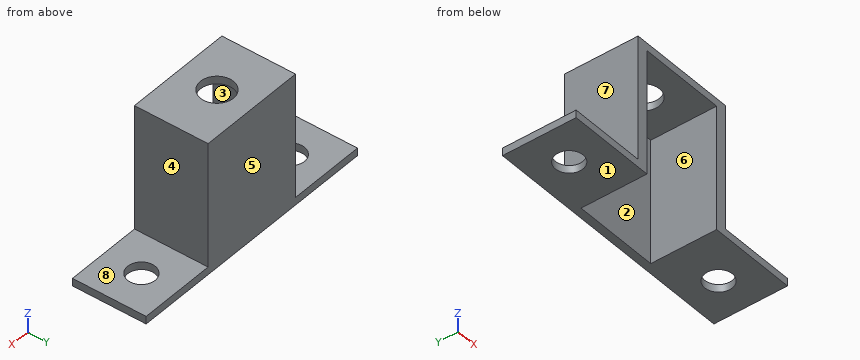
from build123d import *

# Parameters (mm, degrees)
F0_W     = 17.78
F0_H     = 1.778
F1_DEPTH = 17.018
F0_W_2   = 19.9898
F0_H_2   = 28.956
F2_DEPTH = 1.778
F5_R     = 3.175
F4_R     = 3.175
F3_R     = 3.81
F6_DEPTH = 25.4


with BuildPart() as f1:
    # F0 (on Front) → F1 (new body)
    with BuildSketch(Plane.XZ):
        Polygon((-12.296648, -10.522948), (-12.296648, -12.300948), (-9.756648, -12.300948), (-9.756648, 16.655052), (10.233152, 16.655052), (10.233152, -12.300948), (12.773152, -12.300948), (12.773152, -10.522948), (12.773152, 18.433052), (-12.296648, 18.433052), align=None)
        with Locations((-21.186648, -11.411948)):
            Rectangle(F0_W, F0_H)
        with Locations((21.663152, -11.411948)):
            Rectangle(F0_W, F0_H)
    extrude(amount=F1_DEPTH)

    # F0 (on Front) → F2 (join)
    with BuildSketch(Plane.XZ):
        with Locations((0.238252, 2.177052)):
            Rectangle(F0_W_2, F0_H_2)
    extrude(amount=F2_DEPTH)

    # F5 (on face) + F4 (on face) + F3 (on face) → F6 (cut)
    with BuildSketch(Plane.XY.offset(-10.522948)):
        with Locations((21.663152, -8.255)):
            Circle(F5_R)
    with BuildSketch(Plane.XY.offset(-10.522948)):
        with Locations((-21.186648, -8.255)):
            Circle(F4_R)
    with BuildSketch(Plane.XY.offset(18.433052)):
        with Locations((0, -8.251561)):
            Circle(F3_R)
    extrude(amount=-F6_DEPTH, mode=Mode.SUBTRACT)


solid = f1.part
Work out the finished part from the listing and answer in its coordinate system (mm). Face numbers are marked on the shaded views. A direction names the side the tool comes from. Give positions to 0.01 mm unless a question says otherwise; leave off trailing zeros. Loops run counter-clockwise (first coordinate to the right, second up) from the corner with the lowest first, then second, coordinate; pieces in that order, holes last. Notation, with made-up numbers: (-23.5, 23) -> (29.5, 23) arc R15 cw to (29.5, 49) -> close; hole circle Ø3 at (72.25, -33.75). An arc over 180 degrees is marked (long way). Use a Markdown table: item, result. Add a question column.
1. Section A-A on x = 0 is taken. Determine the outline of the cut face in (y, z).
2. Determine the mould class of the marked faces 1, 2, 3 and 4 for opening direction X: released by +X, released by -X, zero draft, split by the parting line, or undercut.
3. Section B-B on y = -10 is taken. Determine the outline of the cut face in (x, z).
4. Flat-ended cylindrical pins translate along their axes: pin 1 Ø3 at (y, z) = (-13.5, 6.5) entering from +X; pin 2 Ø10 at (x, y) = (-21.19, -8.26) entering from +Z; pin 3 Ø4.5 at (y, z) = (-6, -1) entering from -X. Find the tip coordinate at first contact, or state that the pin passes through.
5. For the marked faces 5, 6, 7 and 8, determine the directions among +Z, -Z, +X, -X, +Y, -Y from which every point of the face is accessible in a straight line to the end or side of a thin tool.
6. Section D-D on y = -3.25 is taken. Determine the outline of the cut face in (x, z).
7. Section C-C on z = 10 is taken. Determine the outline of the cut face in (x, y).
8. Find the intervals of material crossed by probe 1 along X at (y, z) = (-10, -7.5); probe 2 along Z at (x, y) = (7.5, -3.5); probe 3 along Z at (x, y) = (25, -2.25), in increasing order.
Results below:
| question | item | result |
|---|---|---|
| 1 | outline | (-17.02, 16.66) -> (-12.06, 16.66) -> (-12.06, 18.43) -> (-17.02, 18.43) -> close; (-4.44, 16.66) -> (-1.78, 16.66) -> (-1.78, -12.3) -> (0, -12.3) -> (0, 18.43) -> (-4.44, 18.43) -> close |
| 2 | face 1 | zero draft |
| 2 | face 2 | undercut |
| 2 | face 3 | undercut |
| 2 | face 4 | released by +X |
| 3 | outline | (-30.08, -12.3) -> (-23.84, -12.3) -> (-23.84, -10.52) -> (-30.08, -10.52) -> close; (-18.53, -12.3) -> (-9.76, -12.3) -> (-9.76, 16.66) -> (-3.39, 16.66) -> (-3.39, 18.43) -> (-12.3, 18.43) -> (-12.3, -10.52) -> (-18.53, -10.52) -> close; (3.39, 16.66) -> (10.23, 16.66) -> (10.23, -12.3) -> (19.01, -12.3) -> (19.01, -10.52) -> (12.77, -10.52) -> (12.77, 18.43) -> (3.39, 18.43) -> close; (24.32, -12.3) -> (30.55, -12.3) -> (30.55, -10.52) -> (24.32, -10.52) -> close |
| 4 | pin 1 | stops at x = 12.77 |
| 4 | pin 2 | stops at z = -10.52 |
| 4 | pin 3 | stops at x = -12.3 |
| 5 | face 5 | +Z, -Z, +X, -X, +Y |
| 5 | face 6 | -Z, -Y |
| 5 | face 7 | +Z, -X, +Y, -Y |
| 5 | face 8 | +Z, +X, +Y, -Y |
| 6 | outline | (-30.08, -12.3) -> (-9.76, -12.3) -> (-9.76, 16.66) -> (10.23, 16.66) -> (10.23, -12.3) -> (30.55, -12.3) -> (30.55, -10.52) -> (12.77, -10.52) -> (12.77, 18.43) -> (-12.3, 18.43) -> (-12.3, -10.52) -> (-30.08, -10.52) -> close |
| 7 | outline | (-12.3, -17.02) -> (-9.76, -17.02) -> (-9.76, -1.78) -> (10.23, -1.78) -> (10.23, -17.02) -> (12.77, -17.02) -> (12.77, 0) -> (-12.3, 0) -> close |
| 8 | probe 1 | x = -12.3 to -9.76, 10.23 to 12.77 |
| 8 | probe 2 | z = 16.66 to 18.43 |
| 8 | probe 3 | z = -12.3 to -10.52 |
